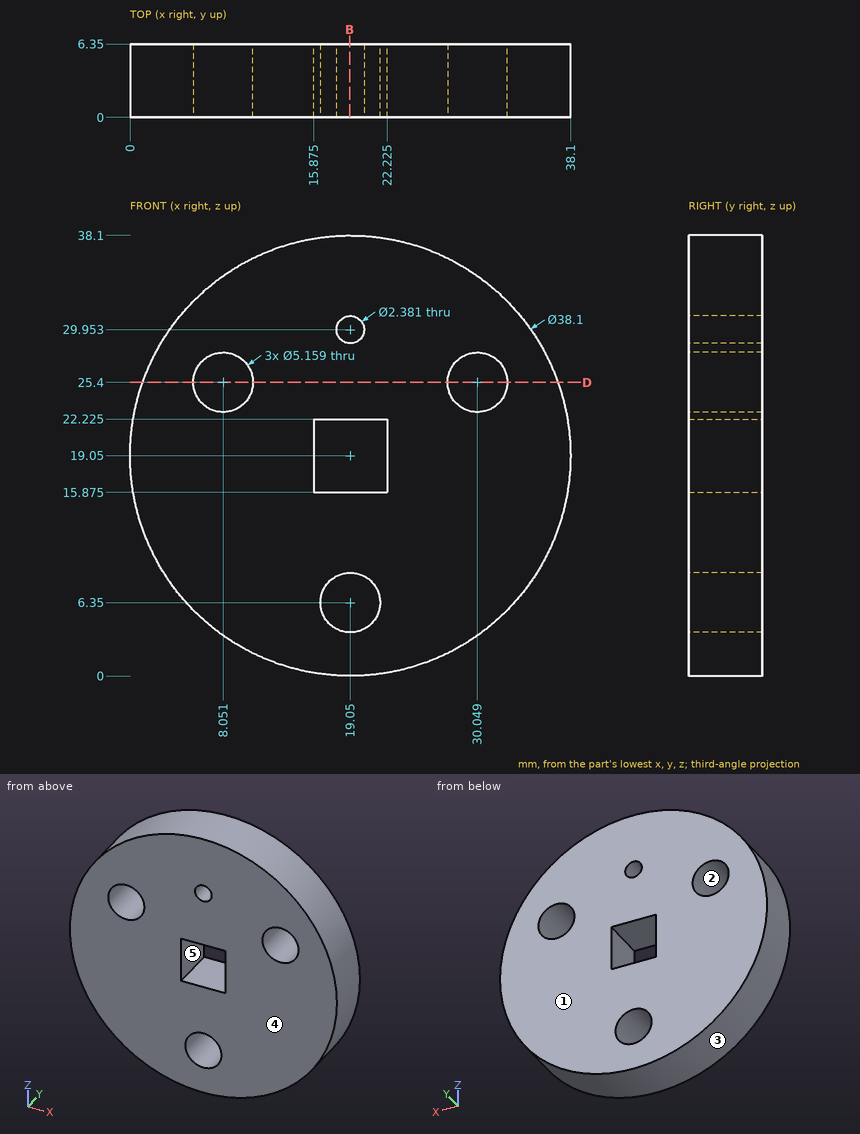
Verification items for this drawing (mm, ordinates from the low corner). A direction names the side the tool comes from. Give positions to 0.01 mm unless a question says otherwise; leave off trailing zeros. Loops run counter-clockwise (first coordinate to the right, second up) from the corner with the lowest first, then second, coordinate; pieces in that order, holes last. Notation, with made-up numbers: M 52.5,-13 L 75.5,-13 A26 ccw 75.5,14 Z; hole C 54,8.25 d10. An arc over 180 degrees is marked long. Answer in a Markdown table with one row per item.
1) Cross-section at B-B (x = 19). Count the separate pieces of the cut face and the enclosed holes in it, plus the area to 3 significant figures.
Solutions:
| item | result |
|---|---|
| separate pieces | 4 |
| enclosed holes | 0 |
| area | 154 mm^2 |
2) Mould release check, pull along Z, two halves, no side actions. Record for the marked faces 1, 2 and 3: released by +Z, released by -Z, zero draft, split by the parting line, or undercut.
Solutions:
| item | result |
|---|---|
| face 1 | zero draft |
| face 2 | undercut |
| face 3 | split by the parting line |
3) Thickness scan on line 1 (Z direction, x = 19.05, y = 2.25) (1 decimal); line 2 (X direction, y = 4, z = 25); line 3 (X direction, y = 4, z = 25.4). Record the ranges inside material, lowest first.
Solutions:
| item | result |
|---|---|
| line 1 | z = 0 to 3.8, 8.9 to 15.9, 22.2 to 28.8, 31.1 to 38.1 |
| line 2 | x = 0.95 to 5.5, 10.6 to 27.5, 32.6 to 37.15 |
| line 3 | x = 1.09 to 5.47, 10.63 to 27.47, 32.63 to 37.01 |
4) Depth check by flat-ended pin: pin 1 (6 mm diameter, centred on x = 8.05, z = 25.4, fed in from -Y); pin 2 (4 mm diameter, centred on x = 30.05, z = 25.4, fed in from +Y); pin 3 (3 mm diameter, centred on y = 5.5, z = 27.5, fed in from -X); pin 4 (3 mm diameter, centred on x = 20, y = 4.5, fed in from +Z). Enter the tip coordinate at first touch or a pass-through.
Solutions:
| item | result |
|---|---|
| pin 1 | stops at y = 0 |
| pin 2 | passes through |
| pin 3 | stops at x = 1.31 |
| pin 4 | stops at z = 38.1 |
5) Tool access check on the marked faces 4 and 5. Record the directions out of +Z, -Z, +X, -X, +Y, -Y that give a thin tool (end or side, any length) a straight path to the whole face; none if there is none.
Solutions:
| item | result |
|---|---|
| face 4 | +Z, -Z, +X, -X, -Y |
| face 5 | +Y, -Y |
6) Cross-section at D-D (z = 25.4). Enter the section's corners in (x, y).
Solutions:
| item | result |
|---|---|
| outline | M 1.09,0 L 5.47,0 L 5.47,6.35 L 1.09,6.35 Z; M 10.63,0 L 27.47,0 L 27.47,6.35 L 10.63,6.35 Z; M 32.63,0 L 37.01,0 L 37.01,6.35 L 32.63,6.35 Z |
